For this review, take the finished solid that the model builds, in its own axes (mm). Coordinates: 2 decimals unless noted, no trailing zeros. Write each loop counter-clockwise with the first axis right and the second up, starting at its lowest first coordinate (ties: lowest second). Pieces come first, ordered by that corner, then holes. Notation, with made-up numbers: (-25.5, 15) -> (15.5, 15) arc R7 ccw to (15.5, 27) -> close; hole circle Ø10 at (75, 73). An arc over 180 degrees is marked (long way). Put each result on its own line as item: value. Start each with the question number.
Item 1: Insertion check: P1, Ø1, axis at x = -11, z = 1.5, coming from the -Y side. The pin has a flat end and moves straight along its axis. Give the tip position at first contact, or say it passes through.
Item 2: Consider section A-A on y = -12. Give the boundary of the cut face in (x, z), and give its area (3 significant figures).
Item 3: Consider section B-B on x = -3. Give the boundary of the cut face in (y, z).
Item 4: Consider section C-C on z = 0.5. Give the number of separate pieces and of enclosed holes in the cut face, and give its area (3 significant figures).
Item 5: To check wall thickness, follow L1, parallel to X at y = -39.5, z = 1.45; L2, parallel to Y at x = 11, z = 1.15; L3, parallel to X at y = -16.5, z = 1.4. State the ranges of each line that lie inside material, in increasing order.
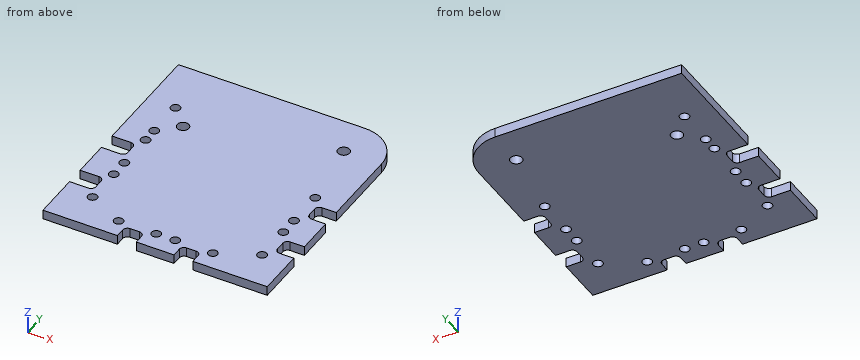
```python
from build123d import *

# Parameters (mm, degrees)
SKETCH_1_R      = 1.25
SKETCH_1_R_2    = 1
EXTRUDE_2_DEPTH = 2


with BuildPart() as part:
    # 草圖1 → 填料-伸長2 (new body)
    with BuildSketch(Plane.XY):
        with BuildLine():
            Line((19.058094933, -28.1179941), (19.058094933, -12.6179941))
            ThreePointArc((19.058094933, -12.6179941), (16.714949182, -6.961139851), (11.058094933, -4.6179941))
            Line((11.058094933, -4.6179941), (-7.541905067, -4.6179941))
            Line((-7.541905067, -4.6179941), (-27.541905067, -4.6179941))
            Line((-27.541905067, -4.6179941), (-28.541905067, -4.6179941))
            Line((-28.541905067, -4.6179941), (-28.541905067, -5.6179941))
            Line((-28.541905067, -5.6179941), (-28.541905067, -12.6179941))
            Line((-28.541905067, -12.6179941), (-28.541905067, -28.1179941))
            Line((-28.541905067, -28.1179941), (-28.541905067, -29.6179941))
            Line((-28.541905067, -29.6179941), (-26.541905067, -29.6179941))
            Line((-26.541905067, -29.6179941), (-24.541905067, -29.6179941))
            ThreePointArc((-24.541905067, -29.6179941), (-23.834798286, -29.910887319), (-23.541905067, -30.6179941))
            Line((-23.541905067, -30.6179941), (-23.541905067, -32.6179941))
            ThreePointArc((-23.541905067, -32.6179941), (-23.834798286, -33.325100881), (-24.541905067, -33.6179941))
            Line((-24.541905067, -33.6179941), (-26.541905067, -33.6179941))
            Line((-26.541905067, -33.6179941), (-28.541905067, -33.6179941))
            Line((-28.541905067, -33.6179941), (-28.541905067, -41.6179941))
            Line((-28.541905067, -41.6179941), (-26.541905067, -41.6179941))
            Line((-26.541905067, -41.6179941), (-24.541905067, -41.6179941))
            ThreePointArc((-24.541905067, -41.6179941), (-23.834798286, -41.910887319), (-23.541905067, -42.6179941))
            Line((-23.541905067, -42.6179941), (-23.541905067, -44.6179941))
            ThreePointArc((-23.541905067, -44.6179941), (-23.834798286, -45.325100881), (-24.541905067, -45.6179941))
            Line((-24.541905067, -45.6179941), (-26.541905067, -45.6179941))
            Line((-26.541905067, -45.6179941), (-28.541905067, -45.6179941))
            Line((-28.541905067, -45.6179941), (-28.541905067, -52.6179941))
            Line((-28.541905067, -52.6179941), (-28.541905067, -53.6179941))
            Line((-28.541905067, -53.6179941), (-28.541905067, -55.6179941))
            Line((-28.541905067, -55.6179941), (-12.741905067, -55.6179941))
            Line((-12.741905067, -55.6179941), (-12.741905067, -53.6179941))
            ThreePointArc((-12.741905067, -53.6179941), (-12.449011848, -52.910887319), (-11.741905067, -52.6179941))
            Line((-11.741905067, -52.6179941), (-9.741905067, -52.6179941))
            ThreePointArc((-9.741905067, -52.6179941), (-9.034798286, -52.910887319), (-8.741905067, -53.6179941))
            Line((-8.741905067, -53.6179941), (-8.741905067, -55.6179941))
            Line((-8.741905067, -55.6179941), (-0.741905067, -55.6179941))
            Line((-0.741905067, -55.6179941), (-0.741905067, -53.6179941))
            ThreePointArc((-0.741905067, -53.6179941), (-0.449011848, -52.910887319), (0.258094933, -52.6179941))
            Line((0.258094933, -52.6179941), (2.258094933, -52.6179941))
            ThreePointArc((2.258094933, -52.6179941), (2.965201714, -52.910887319), (3.258094933, -53.6179941))
            Line((3.258094933, -53.6179941), (3.258094933, -55.6179941))
            Line((3.258094933, -55.6179941), (19.058094933, -55.6179941))
            Line((19.058094933, -55.6179941), (19.058094933, -53.6179941))
            Line((19.058094933, -53.6179941), (19.058094933, -52.6179941))
            Line((19.058094933, -52.6179941), (19.058094933, -45.6179941))
            Line((19.058094933, -45.6179941), (18.039175344, -45.6179941))
            Line((18.039175344, -45.6179941), (16.039175344, -45.6179941))
            ThreePointArc((16.039175344, -45.6179941), (15.332068562, -45.325100881), (15.039175344, -44.6179941))
            Line((15.039175344, -44.6179941), (15.039175344, -42.6179941))
            ThreePointArc((15.039175344, -42.6179941), (15.332068562, -41.910887319), (16.039175344, -41.6179941))
            Line((16.039175344, -41.6179941), (18.039175344, -41.6179941))
            Line((18.039175344, -41.6179941), (19.058094933, -41.6179941))
            Line((19.058094933, -41.6179941), (19.058094933, -33.6179941))
            Line((19.058094933, -33.6179941), (18.039175344, -33.6179941))
            Line((18.039175344, -33.6179941), (16.039175344, -33.6179941))
            ThreePointArc((16.039175344, -33.6179941), (15.332068562, -33.325100881), (15.039175344, -32.6179941))
            Line((15.039175344, -32.6179941), (15.039175344, -30.6179941))
            ThreePointArc((15.039175344, -30.6179941), (15.332068562, -29.910887319), (16.039175344, -29.6179941))
            Line((16.039175344, -29.6179941), (18.039175344, -29.6179941))
            Line((18.039175344, -29.6179941), (19.058094933, -29.6179941))
            Line((19.058094933, -29.6179941), (19.058094933, -28.1179941))
        make_face()
        with Locations((-18.541905067, -20.6179941)):
            Circle(SKETCH_1_R, mode=Mode.SUBTRACT)
        with Locations((-6.741905067, -51.6179941)):
            Circle(SKETCH_1_R_2, mode=Mode.SUBTRACT)
        with Locations((-14.741905067, -51.6179941)):
            Circle(SKETCH_1_R_2, mode=Mode.SUBTRACT)
        with Locations((5.258094933, -51.6179941)):
            Circle(SKETCH_1_R_2, mode=Mode.SUBTRACT)
        with Locations((-22.541905067, -16.3679941)):
            Circle(SKETCH_1_R_2, mode=Mode.SUBTRACT)
        with Locations((-22.541905067, -24.3679941)):
            Circle(SKETCH_1_R_2, mode=Mode.SUBTRACT)
        with Locations((13.458094933, -39.6179941)):
            Circle(SKETCH_1_R_2, mode=Mode.SUBTRACT)
        with Locations((13.458094933, -47.6179941)):
            Circle(SKETCH_1_R_2, mode=Mode.SUBTRACT)
        with Locations((11.058094933, -12.6179941)):
            Circle(SKETCH_1_R, mode=Mode.SUBTRACT)
        with Locations((-22.541905067, -27.6179941)):
            Circle(SKETCH_1_R_2, mode=Mode.SUBTRACT)
        with Locations((-22.541905067, -35.6179941)):
            Circle(SKETCH_1_R_2, mode=Mode.SUBTRACT)
        with Locations((-2.741905067, -51.6179941)):
            Circle(SKETCH_1_R_2, mode=Mode.SUBTRACT)
        with Locations((-22.541905067, -39.6179941)):
            Circle(SKETCH_1_R_2, mode=Mode.SUBTRACT)
        with Locations((-22.541905067, -47.6179941)):
            Circle(SKETCH_1_R_2, mode=Mode.SUBTRACT)
        with Locations((13.458094933, -27.6179941)):
            Circle(SKETCH_1_R_2, mode=Mode.SUBTRACT)
        with Locations((13.458094933, -35.6179941)):
            Circle(SKETCH_1_R_2, mode=Mode.SUBTRACT)
    extrude(amount=EXTRUDE_2_DEPTH)


solid = part.part
```
Return value:
1. P1: y = -52.62
2. outline: (-28.54, 0) -> (9.97, 0) -> (9.97, 2) -> (-28.54, 2) -> close; (12.14, 0) -> (19.03, 0) -> (19.03, 2) -> (12.14, 2) -> close
2. area: 90.8 mm^2
3. outline: (-55.62, 0) -> (-52.58, 0) -> (-52.58, 2) -> (-55.62, 2) -> close; (-50.65, 0) -> (-4.62, 0) -> (-4.62, 2) -> (-50.65, 2) -> close
4. separate pieces: 1
4. enclosed holes: 16
4. area: 2,270 mm^2
5. L1: -28.54 to -23.53, -21.55 to 12.47, 14.45 to 19.06
5. L2: -55.62 to -13.87, -11.37 to -4.62
5. L3: -28.54 to -23.53, -21.55 to 19.06
